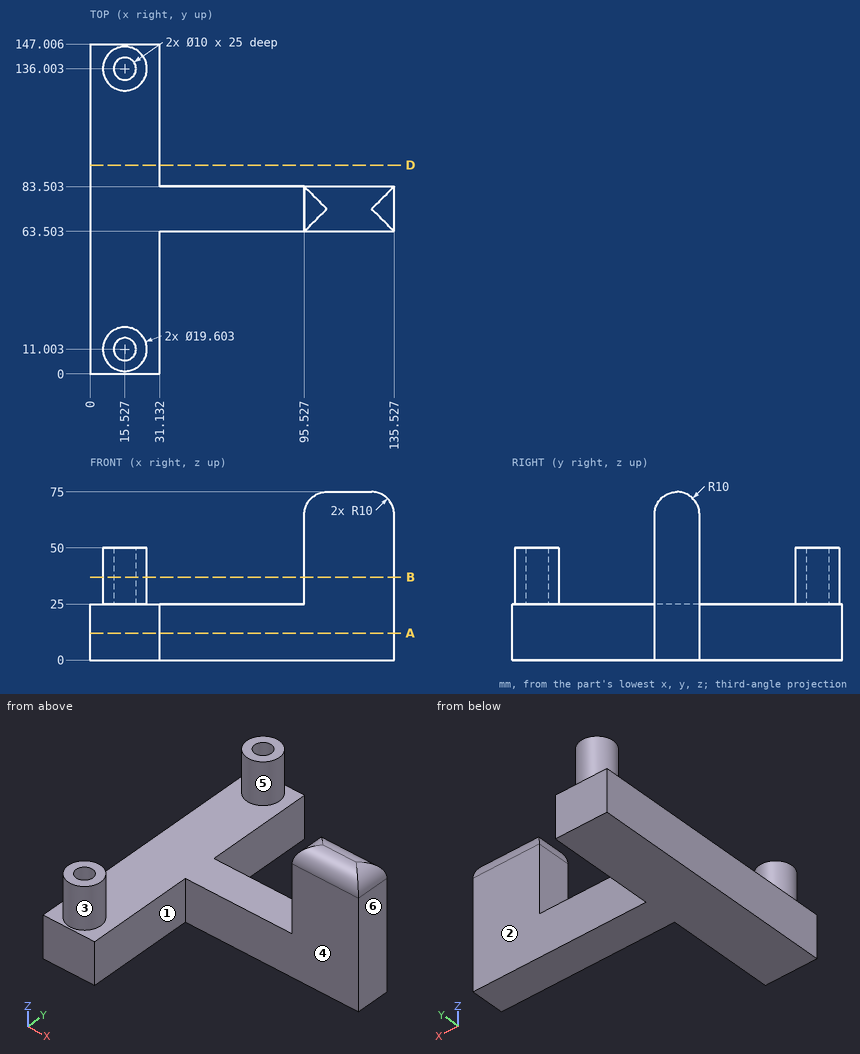
The figure shows three views and two pictorial views of one solid part (mm, origin at its lowest corner). Answer the questions. A direction names the side the tool comes from. Coordinates: 2 decimals unless noted, no trailing zeros. Loops run counter-clockwise (first coordinate to the right, second up) from the corner with the lowest first, then second, coordinate; pieces in that order, holes last. Notation, with made-up numbers: (88, 13) -> (133, 13) arc R11 cw to (133, 17) -> close; hole circle Ø2 at (-11, 7). An arc over 180 degrees is marked (long way). Return JSON: item names as keys, results as strings. Group by question number.
(1) Find the intervals of material crossed by probe 1 along X at (y, z) = (65, 56); probe 2 along X at (y, z) = (93, 6); probe 3 along Y at (x, z) = (108.5, 32.5), in increasing order. Write a range as from..to.
(2) A cutting plane is placed at A-A on z = 12. Write down the section's boundary in (x, y).
(3) A cutting plane is placed at D-D on y = 93. Write down the section's boundary in (x, z), and give its area (3 significant figures).
(4) A cutting plane is placed at B-B on z = 37. Write down the section's boundary in (x, y).
(5) Which of the six approach directions +Z, -Z, +X, -X, +Y, -Y give full straight-line access (tool end or side, diameter ignored) to the marked faces 1, 2 and 3?
(6) Determine the mould class of the marked faces 4, 5 and 6 for opening direction Y: released by +Y, released by -Y, zero draft, split by the parting line, or undercut.
(7) Given pin 1 Ø5 at (x, y) = (15.5, 9.5) entering from +Z; pin 2 Ø6 at (y, z) = (109.5, 29.5) entering from -X; pin 3 Ø8 at (x, y) = (17, 137) entering from +Z; pin 4 Ø12.5 at (y, z) = (28, 13.5) entering from +X, each flat-ended and moving along its own axis, determine where each tip first touches the part or whether it passes through.
The answers:
{
 "1": {"probe 1": "x = 95.53..135.53", "probe 2": "x = 0..31.13", "probe 3": "y = 63.5..83.5"},
 "2": {"outline": "(0, 0) -> (31.13, 0) -> (31.13, 63.5) -> (135.53, 63.5) -> (135.53, 83.5) -> (31.13, 83.5) -> (31.13, 147.01) -> (0, 147.01) -> close"},
 "3": {"outline": "(0, 0) -> (31.13, 0) -> (31.13, 25) -> (0, 25) -> close", "area": "778 mm^2"},
 "4": {"outline": "circle Ø19.6 at (15.53, 11); circle Ø19.6 at (15.53, 136); (95.53, 63.5) -> (135.53, 63.5) -> (135.53, 83.5) -> (95.53, 83.5) -> close; hole circle Ø10 at (15.53, 11); hole circle Ø10 at (15.53, 136)"},
 "5": {"face 1": "+Z, -Z, +X, -Y", "face 2": "+Z, -Z, +X, +Y", "face 3": "+Z"},
 "6": {"face 4": "released by -Y", "face 5": "undercut", "face 6": "zero draft"},
 "7": {"pin 1": "stops at z = 25", "pin 2": "passes through", "pin 3": "stops at z = 50", "pin 4": "stops at x = 31.13"}
}
